from build123d import *

# Parameters (mm, degrees)
ESQUISSE1_W             = 52
ESQUISSE1_H             = 52
ESQUISSE1_R             = 1.5
BOSS_EXTRU_1_DEPTH      = 1.5
ENL_V_MAT_EXTRU_1_DEPTH = 54.73313689
CONG_1_R                = 3


with BuildPart() as part:
    # Esquisse1 → Boss.-Extru.1 (new body)
    with BuildSketch(Plane.XY):
        with Locations((0, 21)):
            Rectangle(ESQUISSE1_W, ESQUISSE1_H)
        with Locations((-21, 0)):
            Circle(ESQUISSE1_R, mode=Mode.SUBTRACT)
        Circle(ESQUISSE1_R, mode=Mode.SUBTRACT)
        with Locations((21, 0)):
            Circle(ESQUISSE1_R, mode=Mode.SUBTRACT)
        with Locations((0, 42)):
            Circle(ESQUISSE1_R, mode=Mode.SUBTRACT)
        with Locations((0, 21)):
            Circle(ESQUISSE1_R, mode=Mode.SUBTRACT)
    extrude(amount=BOSS_EXTRU_1_DEPTH)

    # Esquisse2 → Enlèv. mat.-Extru.1 (cut, through all)
    with BuildSketch(Plane.XY.offset(1.5)):
        Polygon((-26, 47), (-5, 47), (-26, 5), align=None)
        Polygon((26, 47), (26, 5), (5, 47), align=None)
    extrude(amount=-ENL_V_MAT_EXTRU_1_DEPTH, mode=Mode.SUBTRACT)

    # Congé1
    cong_1_edges = [part.edges().sort_by_distance(p)[0] for p in [
        (-26, 5, 0.75),
        (-5, 47, 0.75),
        (5, 47, 0.75),
        (26, 5, 0.75),
        (26, -5, 0.75),
        (-26, -5, 0.75),
    ]]
    fillet(cong_1_edges, radius=CONG_1_R)


solid = part.part
Work out the finished part from the listing and answer in its coordinate system (mm). Give positions to 0.01 mm unless a question says otherwise; leave off trailing zeros. Loops run counter-clockwise (first coordinate to the right, second up) from the corner with the lowest first, then second, coordinate; pieces in that order, holes last. Notation, with made-up numbers: (14.25, 72) -> (29.25, 72) arc R13 ccw to (29.25, 85) -> close; hole circle Ø2 at (50, 45.5). An arc over 180 degrees is marked (long way). Use a Markdown table: item, result. Add a question column.
1. Determine the mould class of faces 1 (the cylindrical face through (-25.14, -4.1, 0.76)), 2 (the cylindrical face through (-0.325, 40.536, 0.74)), 3 (the flat face through (0, 47, 1)), 4 (the flat face through (26, 1, 1)) for opening direction X: released by +X, released by -X, zero draft, split by the parting line, or undercut.
2. Flat-ended cylindrical pins translate along their axes: pin 1 Ø2.5 at (x, y) = (0, 0) entering from -Z; pin 2 Ø6 at (x, y) = (-19, 23.5) entering from +Z. Find the tip coordinate at first contact, or state that the pin passes through.
3. Section B-B on x = 21 is taken. Determine the outline of the cut face in (y, z), and give its area (3 significant figures).
4. Section D-D on y = 9.5 is taken. Determine the outline of the cut face in (x, z).
5. Section C-C on z = 0.3 is taken. Determine the outline of the cut face in (x, y).
6. Find the intervals of material crossed by probe 1 along Y at (x, z) = (0, 0.5); probe 2 along Y at (x, z) = (-21, 0.3); probe 3 along X at (y, z) = (18, 0.6), in increasing order.
7. Section A-A on y = 42 is taken. Determine the outline of the cut face in (x, z).
Results below:
| question | item | result |
|---|---|---|
| 1 | face 1 | released by -X |
| 1 | face 2 | undercut |
| 1 | face 3 | zero draft |
| 1 | face 4 | released by +X |
| 2 | pin 1 | passes through |
| 2 | pin 2 | stops at z = 1.5 |
| 3 | outline | (-5, 0) -> (-1.5, 0) -> (-1.5, 1.5) -> (-5, 1.5) -> close; (1.5, 0) -> (15, 0) -> (15, 1.5) -> (1.5, 1.5) -> close |
| 3 | area | 25.5 mm^2 |
| 4 | outline | (-23.75, 0) -> (23.75, 0) -> (23.75, 1.5) -> (-23.75, 1.5) -> close |
| 5 | outline | (-26, -2) arc R3 ccw to (-23, -5) -> (23, -5) arc R3 ccw to (26, -2) -> (26, 4.29) arc R3 ccw to (25.68, 5.63) -> (5.83, 45.34) arc R3 ccw to (3.15, 47) -> (-3.15, 47) arc R3 ccw to (-5.83, 45.34) -> (-25.68, 5.63) arc R3 ccw to (-26, 4.29) -> close; hole circle Ø3 at (-21, 0); hole circle Ø3 at (0, 0); hole circle Ø3 at (0, 21); hole circle Ø3 at (0, 42); hole circle Ø3 at (21, 0) |
| 6 | probe 1 | y = -5 to -1.5, 1.5 to 19.5, 22.5 to 40.5, 43.5 to 47 |
| 6 | probe 2 | y = -5 to -1.5, 1.5 to 15 |
| 6 | probe 3 | x = -19.5 to 19.5 |
| 7 | outline | (-7.5, 0) -> (-1.5, 0) -> (-1.5, 1.5) -> (-7.5, 1.5) -> close; (1.5, 0) -> (7.5, 0) -> (7.5, 1.5) -> (1.5, 1.5) -> close |
